from build123d import *

# Parameters (mm, degrees)
F0_R     = 7.9375
F0_R_2   = 4.7625
F1_DEPTH = 25.4
F2_SIZE  = 1.5875
F3_W     = 5.55625
F3_H     = 19.05
F5_SIZE  = 0.79374


# Not quite as in the source:
# - a fillet or chamfer is up to 0.001 mm smaller than in the source, because OpenCascade refuses the exact size


with BuildPart() as f1:
    # F0 (on Top) → F1 (new body)
    with BuildSketch(Plane.XY):
        Circle(F0_R)
        Circle(F0_R_2, mode=Mode.SUBTRACT)
    extrude(amount=F1_DEPTH)

    # F2
    f2_edges = [f1.edges().sort_by_distance(p)[0] for p in [
        (-7.9375, 0, 25.4),
    ]]
    chamfer(f2_edges, length=F2_SIZE)

    # F3 (on Front) → F4 (revolve, cut)
    with BuildSketch(Plane.XZ):
        with Locations((2.778125, 12.7)):
            Rectangle(F3_W, F3_H)
    revolve(axis=Axis((0, 0, 0), (0, 0, -1)), mode=Mode.SUBTRACT)

    # F5 (size 0.79375 in the source; OpenCascade refuses exactly that, so slightly less here)
    f5_edges = [f1.edges().sort_by_distance(p)[0] for p in [
        (-4.7625, 0, 0),
        (-4.7625, 0, 3.175),
        (-4.7625, 0, 22.225),
        (-4.7625, 0, 25.4),
    ]]
    chamfer(f5_edges, length=F5_SIZE)


solid = f1.part
Check sheet for the modelled part. Datum: model origin and axes. Units: mm. A direction names the side the tool comes from. Give positions to 0.01 mm unless a question says otherwise; leave off trailing zeros. Order: outer loops, then holes, each group sorted by start corner. A loop starts at its lowest first (then second) coordinate and runs counter-clockwise, first axis right, second up. Notation, with made-up numbers: (60, 13.25) - (90, 13.25) arc R17 ccw to (90, 33.25) - close; hole circle Ø9 at (-6.5, -33). An arc over 180 degrees is marked (long way). Answer as CSV lines item,"result".
1. Mould release check, pull along X, two halves, no side actions. Record for faces 3 (the face through (-3.78, -2.9, 1.58)), 4 (the face through (0, -6, 25.4)), 5 (the face through (-1.72, -7.75, 11.74)): released by +X, released by -X, zero draft, split by the parting line, or undercut.
Result sheet:
face 3,"undercut"
face 4,"zero draft"
face 5,"split by the parting line"
2. Tool access check on faces 1 (the face through (-3.78, -2.9, 23.8)), 2 (the face through (5.3, -1.67, 12.83)). Record the directions out of +Z, -Z, +X, -X, +Y, -Y that give a thin tool (end or side, any length) a straight path to the whole face; none if there is none.
Result sheet:
face 1,"+Z, -Z"
face 2,"none"
3. Section check C-C (z = 6). Record the boundary of the cut face in (x, y) (1 decimal).
Result sheet:
outline,"circle Ø15.9 at (0, 0); hole circle Ø11.1 at (0, 0)"
4. Go/stop test with flat-tipped pins: P1, Ø1.5, axis at y = 4.5, z = 18, coming from the +X side; P2, Ø8, axis at y = -3, z = 4, coming from the -X side; P3, Ø5, axis at y = 4, z = 21, coming from the +X side; P4, Ø1, axis at y = -1, z = 21, coming from the +X side. Record where each tip stops, or that it passes through.
Result sheet:
P1,"x = 7"
P2,"x = -7.94"
P3,"x = 7.79"
P4,"x = 7.92"
5. Scan lines: probe 1 along Y at (x, z) = (0, 17.25); probe 2 along Y at (x, z) = (0, 1.9); probe 3 along X at (y, z) = (-3.25, 1.75). Record each from-to range of solid material in increasing order. Write a range as from..to.
Result sheet:
probe 1,"-7.94..-5.56, 5.56..7.94"
probe 2,"-7.94..-4.76, 4.76..7.94"
probe 3,"-7.24..-3.48, 3.48..7.24"
